from build123d import *

# Parameters (mm, degrees)
SKETCH_2_W        = 250
SKETCH_2_H        = 8
EXTRUDE_262_DEPTH = 15
HOLE_WIZARD_6_D   = 6
CHAMFER_1283_SIZE = 4


with BuildPart() as part:
    # Эскиз2 → Extrude 262 (new body)
    with BuildSketch(Plane.XY):
        Rectangle(SKETCH_2_W, SKETCH_2_H)
    extrude(amount=-EXTRUDE_262_DEPTH)

    # Отверстия-6мм (through all)
    with Locations(Plane(origin=(0, 4, 0), x_dir=(-1, 0, 0), z_dir=(0, 1, 0))):
        with Locations((90, -7.5), (-90, -7.5), (30, -7.5), (-30, -7.5)):
            Hole(HOLE_WIZARD_6_D / 2)

    # Chamfer 1283
    chamfer_1283_edges = [part.edges().sort_by_distance(p)[0] for p in [
        (125, -4, -7.5),
        (-125, -4, -7.5),
    ]]
    chamfer(chamfer_1283_edges, length=CHAMFER_1283_SIZE)


solid = part.part
Input: part model. Units: mm. Frame: model coordinates. Give positions to 0.01 mm unless a question says otherwise; leave off trailing zeros. Order: outer loops, then holes, each group sorted by start corner. A loop starts at its lowest first (then second) coordinate and runs counter-clockwise, first axis right, second up.
Q1. Section B-B on z = -7.5. Output: boundary loops of the cut face in (x, y), and give its area (3 significant figures).
Checked values:
outline: (-125, 0) - (-121, -4) - (-93, -4) - (-93, 4) - (-125, 4) - close; (-87, -4) - (-33, -4) - (-33, 4) - (-87, 4) - close; (-27, -4) - (27, -4) - (27, 4) - (-27, 4) - close; (33, -4) - (87, -4) - (87, 4) - (33, 4) - close; (93, -4) - (121, -4) - (125, 0) - (125, 4) - (93, 4) - close
area: 1,790 mm2
Q2. Section A-A on y = -1.5. Output: boundary loops of the cut face in (x, z).
Checked values:
outline: (-123.5, -15) - (123.5, -15) - (123.5, 0) - (-123.5, 0) - close; hole circle Ø6 at (-90, -7.5); hole circle Ø6 at (-30, -7.5); hole circle Ø6 at (30, -7.5); hole circle Ø6 at (90, -7.5)
Q3. Section C-C on x = -30. Output: boundary loops of the cut face in (y, z), and give its area (3 significant figures).
Checked values:
outline: (-4, -15) - (4, -15) - (4, -10.5) - (-4, -10.5) - close; (-4, -4.5) - (4, -4.5) - (4, 0) - (-4, 0) - close
area: 72.0 mm2
Q4. Ray query, probe 1 along X at (y, z) = (1.75, -7); probe 2 along Z at (x, y) = (-90, 2.5); probe 3 along X at (y, z) = (3.5, -9). Return the intervals inside material, ascending.
Checked values:
probe 1: x = -125 to -92.96, -87.04 to -32.96, -27.04 to 27.04, 32.96 to 87.04, 92.96 to 125
probe 2: z = -15 to -10.5, -4.5 to 0
probe 3: x = -125 to -92.6, -87.4 to -32.6, -27.4 to 27.4, 32.6 to 87.4, 92.6 to 125
